Part model, mm, in its own coordinate system. Face numbers are marked on the shaded views. A direction names the side the tool comes from. Give positions to 0.01 mm unless a question says otherwise; leave off trailing zeros. Write each loop counter-clockwise with the first axis right and the second up, starting at its lowest first coordinate (ties: lowest second). Pieces come first, ordered by that corner, then holes. Notation, with made-up numbers: M 12.25,11 L 56.25,11 A9 cw 56.25,21 Z; hole C -17,75.5 d5. An arc over 180 degrees is marked long. Answer as CSV lines item,"result". Start each with the question number.
Item 1: Pin check, flat tips, straight feed: pin 1 (11 mm diameter, centred on y = 30, z = -5, fed in from +X); pin 2 (17 mm diameter, centred on x = -8.5, y = 29.5, fed in from +Z); pin 3 (1 mm diameter, centred on y = 27, z = 3.5, fed in from -X); pin 4 (3.5 mm diameter, centred on x = -20.48, z = -8.75, fed in from -Y). Stop position of each tip, or through.
Item 2: 3-axis set-ups, long thin cutter, end or side, ignore diameter. For the marked faces 1 and 2: which of +Z, -Z, +X, -X, +Y, -Y reach the whole face in a straight line?
Item 3: Band-saw the part on A-A, the plane z = -16.25. List the corners of the cut face in (x, y).
Item 4: Band-saw the part on B-B, the plane z = -8.75. List the corners of the cut face in (x, y), then the cut area to 3 significant figures.
Item 5: Band-saw the part on C-C, the plane x = -58. List the corners of the cut face in (y, z).
Item 6: Band-saw the part on D-D, the plane y = 27.5. Count the separate pieces of the cut face and the enclosed holes in it, then the cut area to 3 significant figures.
Item 7: Wall check: L1, parallel to X at y = 1.95, z = -8.75; L2, parallel to X at y = 1, z = -16; L3, parallel to X at y = 1.1, z = -16.25. Give the ranges that are in metal, low to high. Write a range as from..to.
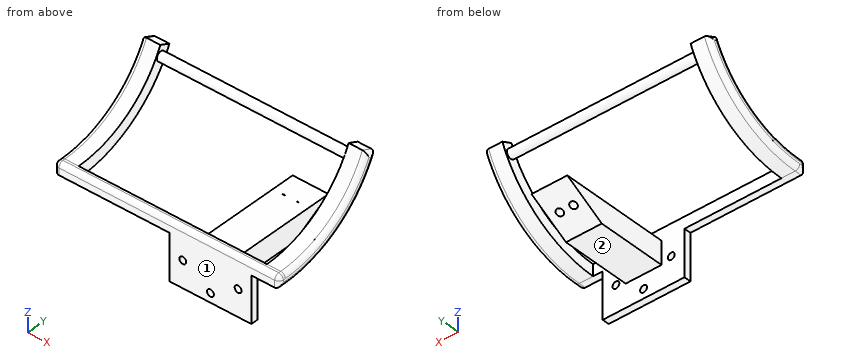
from build123d import *

# Parameters (mm, degrees)
SKETCH1_W           = 17.805
SKETCH1_H           = 20
SKETCH1_W_2         = 38
SKETCH1_H_2         = 5
BOSS_EXTRUDE1_DEPTH = 3
SKETCH3_R           = 1.5
CUT_EXTRUDE1_DEPTH  = 5
SKETCH7_W           = 15.61
SKETCH7_H           = 10
BOSS_EXTRUDE4_DEPTH = 30
BOSS_EXTRUDE5_DEPTH = 15.61
SKETCH9_R           = 1.5
CUT_EXTRUDE2_DEPTH  = 5
BOSS_EXTRUDE6_DEPTH = 8
FILLET4_R           = 2
SKETCH10_R          = 2
BOSS_EXTRUDE7_DEPTH = 82


with BuildPart() as part:
    # Sketch1 → Boss-Extrude1 (new body)
    with BuildSketch(Plane(origin=(0, 0, 0), x_dir=(1, 0, 0), z_dir=(0, 1, 0))):
        Polygon((9.368218391, 0.25), (-8.436781609, 0.25), (-26.241781609, 0.25), (-38.436781609, 0.25), (-38.436781609, -4.75), (21.563218391, -4.75), (21.563218391, 0.25), align=None)
        with Locations((0.465718391, 10.25)):
            Rectangle(SKETCH1_W, SKETCH1_H)
        with Locations((-17.339281609, 10.25)):
            Rectangle(SKETCH1_W, SKETCH1_H)
        with Locations((-57.436781609, -2.25)):
            Rectangle(SKETCH1_W_2, SKETCH1_H_2)
    extrude(amount=BOSS_EXTRUDE1_DEPTH)

    # Sketch3 → Cut-Extrude1 (cut)
    with BuildSketch(Plane.XZ):
        with Locations(Location((-20.484687418, -8.75, 0), (0, 0, 270))):
            Circle(SKETCH3_R)
        with Locations(Location((-8.434877213, -16.25, 0), (0, 0, 270))):
            Circle(SKETCH3_R)
        with Locations(Location((3.614932992, -8.75, 0), (0, 0, 270))):
            Circle(SKETCH3_R)
    extrude(amount=-CUT_EXTRUDE1_DEPTH, mode=Mode.SUBTRACT)

    # Sketch7 → Boss-Extrude4 (add)
    with BuildSketch(Plane(origin=(0, 3, 0), x_dir=(1, 0, 0), z_dir=(0, 1, 0))):
        with Locations((-8.436781609, 5.25)):
            Rectangle(SKETCH7_W, SKETCH7_H)
    extrude(amount=BOSS_EXTRUDE4_DEPTH)

    # Sketch8 → Boss-Extrude5 (add)
    with BuildSketch(Plane.ZY.offset(16.241781609)):
        Polygon((-10.25, 33), (-0.25, 50.320508076), (-0.25, 33), align=None)
    extrude(amount=-BOSS_EXTRUDE5_DEPTH)

    # Sketch9 → Cut-Extrude2 (cut)
    with BuildSketch(Plane(origin=(0, 12.688380194, -21.976919162), x_dir=(1, 0, 0), z_dir=(0, 0.4999999999999978, -0.8660254037844399))):
        with Locations(Location((-11.436781609, -33.453838325, 0), (0, 0, 270))):
            Circle(SKETCH9_R)
        with Locations(Location((-5.436781609, -33.453838325, 0), (0, 0, 270))):
            Circle(SKETCH9_R)
    extrude(amount=-CUT_EXTRUDE2_DEPTH, mode=Mode.SUBTRACT)

    # Sketch2 → Boss-Extrude6 (add)
    with BuildSketch(Plane(origin=(21.563218391, 0, 0), x_dir=(0, 0, -1), z_dir=(1, 0, 0))):
        with BuildLine():
            Line((-29.267799241, 48.612273042), (-31.316019317, 44.051045738))
            ThreePointArc((-31.316019317, 44.051045738), (-11.97084483, 27.448628481), (-4.75, 3))
            Line((-4.75, 3), (0.25, 3))
            ThreePointArc((0.25, 3), (-7.773160922, 30.165142757), (-29.267799241, 48.612273042))
        make_face()
    boss_extrude6 = extrude(amount=-BOSS_EXTRUDE6_DEPTH)

    # Mirror1: Boss-Extrude6 across plane
    add(boss_extrude6.mirror(Plane.ZY.offset(27.436781609)))

    # Fillet4
    fillet4_edges = [part.edges().sort_by_distance(p)[0] for p in [
        (-76.436781609, 27.448628481, 11.97084483),
        (-76.436781609, 30.165142757, 7.773160922),
        (-76.436781609, 46.33165939, 30.291909279),
        (21.563218391, 0, 2.25),
        (21.563218391, 1.5, 4.75),
        (21.563218391, 1.5, -0.25),
        (-76.436781609, 1.5, -0.25),
        (-76.436781609, 1.5, 4.75),
        (-76.436781609, 0, 2.25),
        (21.563218391, 27.448628481, 11.97084483),
        (-27.436781609, 0, 4.75),
        (21.563218391, 30.165142757, 7.773160922),
        (21.563218391, 46.33165939, 30.291909279),
    ]]
    fillet(fillet4_edges, radius=FILLET4_R)

    # Sketch10 → Boss-Extrude7 (add)
    with BuildSketch(Plane(origin=(-68.436781609, 0, 0), x_dir=(0, 0, -1), z_dir=(1, 0, 0))):
        with Locations(Location((-26.603637459, 44.285402207, 0), (0, 0, 180))):
            Circle(SKETCH10_R)
    extrude(amount=BOSS_EXTRUDE7_DEPTH)


solid = part.part
Output:
1,pin 1,"x = -0.63"
1,pin 2,"z = -0.25"
1,pin 3,"through"
1,pin 4,"y = 0"
2,face 1,"+Z, -Z, +X, -X, -Y"
2,face 2,"-Z, +X, -X, +Y"
3,outline,"M -26.24,0 L -9.93,0 L -9.93,3 L -26.24,3 Z; M -6.93,0 L 9.37,0 L 9.37,3 L -6.93,3 Z"
4,outline,"M -26.24,0 L -21.98,0 L -21.98,3 L -26.24,3 Z; M -18.98,0 L 2.11,0 L 2.11,3 L -0.63,3 L -0.63,35.6 L -16.24,35.6 L -16.24,3 L -18.98,3 Z; M 5.11,0 L 9.37,0 L 9.37,3 L 5.11,3 Z"
4,area,"598 mm²"
5,outline,"M 0,-0.25 L 3,-0.25 L 3,4.75 L 2,4.75 A2 ccw 0,2.75 Z; C 44.29,26.6 d4"
6,separate pieces,"3"
6,enclosed holes,"0"
6,area,"246 mm²"
7,L1,"-26.24..-21.98, -18.98..2.11, 5.11..9.37"
7,L2,"-26.24..-9.91, -6.96..9.37"
7,L3,"-26.24..-9.93, -6.93..9.37"
